Geometry: final body of the model. Coordinates: model frame, mm. Round coordinates to 2 decimals unless told otherwise and drop trailing zeros. Write each loop counter-clockwise with the first axis right and the second up, starting at its lowest first coordinate (ties: lowest second). Pieces come first, ordered by that corner, then holes.
from build123d import *

# Parameters (mm, degrees)
CUT_EXTRUDE1_START         = 5.842
SKETCH4_R                  = 1.0922
CUT_EXTRUDE1_DEPTH         = 0.508
F_2_56_TAPPED_HOLE2_REACH  = 14.539
F_2_56_TAPPED_HOLE2_BORE_R = 0.889


with BuildPart() as part:
    # Sketch1 → Revolve1 (revolve)
    with BuildSketch(Plane(origin=(0, 0, 0), x_dir=(0, 0, -1), z_dir=(1, 0, 0)), mode=Mode.PRIVATE) as revolve1_sk:
        Polygon((-3.1, 5), (-3.1, 2.925), (-2.6, 2.425), (2.6, 2.425), (3.1, 2.925), (3.1, 5), (2.6, 5.5), (-2.6, 5.5), align=None)
    revolve(revolve1_sk.sketch.rotate(Axis((0, 0, 0), (0, 0, -1)), 90), axis=Axis((0, 0, 0), (0, 0, -1)))

    # Sketch4 → Cut-Extrude1 (cut)
    with BuildSketch(Plane(origin=(0, 0, 0), x_dir=(0, 0, -1), z_dir=(1, 0, 0)).offset(CUT_EXTRUDE1_START)):
        Circle(SKETCH4_R)
    extrude(amount=-CUT_EXTRUDE1_DEPTH, mode=Mode.SUBTRACT)

    # #2-56 Tapped Hole2 bore → #2-56 Tapped Hole2 (cut, up to next)
    with BuildSketch(Plane(origin=(5.334, 0, 0), x_dir=(0, 0, -1), z_dir=(1, 0, 0)), mode=Mode.PRIVATE) as f_2_56_tapped_hole2_sk1:
        Circle(F_2_56_TAPPED_HOLE2_BORE_R)
    f_2_56_tapped_hole2_tool1 = extrude(f_2_56_tapped_hole2_sk1.sketch, amount=-F_2_56_TAPPED_HOLE2_REACH, mode=Mode.PRIVATE) & part.part
    add(f_2_56_tapped_hole2_tool1.solids().sort_by_distance((5.334, 0, 0))[0], mode=Mode.SUBTRACT)


solid = part.part
1) Section A-A on x = 0. Output: boundary loops of the cut face in (y, z) (3 decimals), plus the area to 3 significant figures.
2) Section D-D on z = 0. Output: boundary loops of the cut face in (x, y) (3 decimals).
3) Line query: probe 1 along Y at (x, z) = (0, 1.5) (3 decimals); probe 2 along X at (y, z) = (-1.5, 1). Output: solid intervals per line, ascending.
4) Section B-B on z = -0.75. Output: boundary loops of the cut face in (x, y) (3 decimals).
5) First-contact query: P1, Ø1, axis at x = 1.5, y = 1, coming from the +Z side; P2, Ø2, axis at x = 1.5, y = -0.5, coming from the -Z side; P3, Ø3, axis at y = -2.5, z = 1.5, coming from the -X side. Flat tips, straight axial feed; report the tip coordinate or a pass-through.
6) Draft query along X for faces 1 (the cylindrical face through (-2.423, -0.107, -0.036)), 2 (the cylindrical face through (-1.19, 5.37, 0.04)), 3 (the cylindrical face through (3.82, -0.87, 0.19)). Return one class per face: pulls with the +X half, pulls with the -X half, needs draft (parallel to the pull), parting line crosses it, or undercut.
7) Section C-C on y = 0.25. State how many separate pieces and enclosed holes the cut face has, plus the area to 3 significant figures.
Filled in:
1. outline: (-5.5, -2.6) - (-5, -3.1) - (-2.925, -3.1) - (-2.425, -2.6) - (-2.425, 2.6) - (-2.925, 3.1) - (-5, 3.1) - (-5.5, 2.6) - close; (2.425, -2.6) - (2.925, -3.1) - (5, -3.1) - (5.5, -2.6) - (5.5, 2.6) - (5, 3.1) - (2.925, 3.1) - (2.425, 2.6) - close
1. area: 37.1 mm2
2. outline: (2.256, -0.889) arc R2.425 cw (long way) to (2.256, 0.889) - (5.334, 0.889) - (5.334, 1.092) - (5.39, 1.092) arc R5.5 ccw (long way) to (5.39, -1.092) - (5.334, -1.092) - (5.334, -0.889) - close
3. probe 1: y = -5.5 to -2.425, 2.425 to 5.5
3. probe 2: x = -5.29 to -1.91, 1.91 to 5.29
4. outline: (2.378, -0.477) arc R2.425 cw (long way) to (2.378, 0.477) - (5.334, 0.477) - (5.334, 0.794) - (5.442, 0.794) arc R5.5 ccw (long way) to (5.442, -0.794) - (5.334, -0.794) - (5.334, -0.477) - close
5. P1: passes through
5. P2: stops at z = -2.76
5. P3: stops at x = -5.41
6. face 1: undercut
6. face 2: parting line crosses it
6. face 3: needs draft
7. separate pieces: 3
7. enclosed holes: 0
7. area: 31.9 mm2
